from build123d import *

# Parameters (mm, degrees)
SKETCH1_W                    = 179.07
SKETCH1_H                    = 89.916
BOSS_EXTRUDE1_DEPTH          = 1.651
F_30_0_1285_DIAMETER_HOLE1_D = 3.2639
SKETCH4_W                    = 14.8844
SKETCH4_H                    = 18.8214
BOSS_EXTRUDE2_DEPTH          = 15.6718
LPATTERN1_COUNT              = 8
LPATTERN1_PITCH              = 16.4592
LPATTERN1_COUNT_DIR2         = 2
LPATTERN1_PITCH_DIR2         = 44.958
SKETCH5_W                    = 29.972
SKETCH5_H                    = 6.858
BOSS_EXTRUDE3_DEPTH          = 10.16
LPATTERN2_COUNT              = 4
LPATTERN2_PITCH              = 33.02
LPATTERN2_COUNT_DIR2         = 2
LPATTERN2_PITCH_DIR2         = 74.93
SKETCH6_W                    = 7.62
SKETCH6_H                    = 12.452922763
BOSS_EXTRUDE4_DEPTH          = 10.16
SKETCH7_W                    = 5.08
SKETCH7_H                    = 25.4
BOSS_EXTRUDE5_DEPTH          = 2.54
SKETCH8_W                    = 0.508
SKETCH8_H                    = 0.508
BOSS_EXTRUDE6_DEPTH          = 5.08
LPATTERN3_COUNT              = 10
LPATTERN3_PITCH              = 2.54
LPATTERN3_COUNT_DIR2         = 2
LPATTERN3_PITCH_DIR2         = 2.54


with BuildPart() as part:
    # Sketch1 → Boss-Extrude1 (new body)
    with BuildSketch(Plane(origin=(0, 0, 0), x_dir=(1, 0, 0), z_dir=(0, 1, 0))):
        Rectangle(SKETCH1_W, SKETCH1_H)
    extrude(amount=BOSS_EXTRUDE1_DEPTH)

    # #30 (0.1285) Diameter Hole1 (through all)
    with Locations(Plane(origin=(-85.725, 1.651, 41.021), x_dir=(0, 0, 1), z_dir=(0, 1, 0))):
        with Locations((0, 0), (-82.042, 0), (-82.042, 171.45), (0, 171.45)):
            Hole(F_30_0_1285_DIAMETER_HOLE1_D / 2)

    # Sketch4 → Boss-Extrude2 (add)
    with BuildSketch(Plane(origin=(0, 1.651, 0), x_dir=(1, 0, 0), z_dir=(0, 1, 0))):
        with Locations((-77.7494, -23.3553)):
            Rectangle(SKETCH4_W, SKETCH4_H)
    boss_extrude2 = extrude(amount=BOSS_EXTRUDE2_DEPTH)

    # LPattern1: Boss-Extrude2 8 × 2
    with Locations(*[(i * LPATTERN1_PITCH, 0, -j * LPATTERN1_PITCH_DIR2) for i in range(LPATTERN1_COUNT) for j in range(LPATTERN1_COUNT_DIR2) if (i, j) != (0, 0)]):
        add(boss_extrude2)

    # Sketch5 → Boss-Extrude3 (add)
    with BuildSketch(Plane(origin=(0, 1.651, 0), x_dir=(1, 0, 0), z_dir=(0, 1, 0))):
        with Locations((-67.945, -37.3634)):
            Rectangle(SKETCH5_W, SKETCH5_H)
    boss_extrude3 = extrude(amount=BOSS_EXTRUDE3_DEPTH)

    # LPattern2: Boss-Extrude3 4 × 2
    with Locations(*[(i * LPATTERN2_PITCH, 0, -j * LPATTERN2_PITCH_DIR2) for i in range(LPATTERN2_COUNT) for j in range(LPATTERN2_COUNT_DIR2) if (i, j) != (0, 0)]):
        add(boss_extrude3)

    # Sketch6 → Boss-Extrude4 (add)
    with BuildSketch(Plane(origin=(0, 1.651, 0), x_dir=(1, 0, 0), z_dir=(0, 1, 0))):
        with Locations((84.455, 18.157538618)):
            Rectangle(SKETCH6_W, SKETCH6_H)
    extrude(amount=BOSS_EXTRUDE4_DEPTH)

    # Sketch7 → Boss-Extrude5 (add)
    with BuildSketch(Plane(origin=(0, 1.651, 0), x_dir=(1, 0, 0), z_dir=(0, 1, 0))):
        with Locations((84.455, -4.318)):
            Rectangle(SKETCH7_W, SKETCH7_H)
    extrude(amount=BOSS_EXTRUDE5_DEPTH)

    # Sketch8 → Boss-Extrude6 (add)
    with BuildSketch(Plane(origin=(0, 4.191, 0), x_dir=(1, 0, 0), z_dir=(0, 1, 0))):
        with Locations((85.725, 7.112)):
            Rectangle(SKETCH8_W, SKETCH8_H)
    boss_extrude6 = extrude(amount=BOSS_EXTRUDE6_DEPTH)

    # LPattern3: Boss-Extrude6 10 × 2
    with Locations(*[(-j * LPATTERN3_PITCH_DIR2, 0, i * LPATTERN3_PITCH) for i in range(LPATTERN3_COUNT) for j in range(LPATTERN3_COUNT_DIR2) if (i, j) != (0, 0)]):
        add(boss_extrude6)


solid = part.part
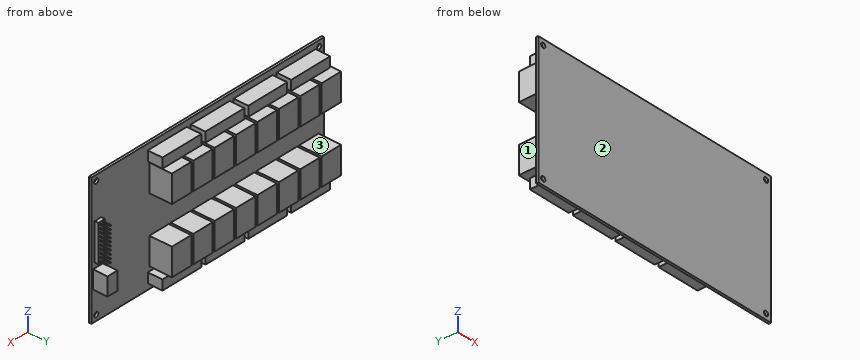
For this review, take the finished solid that the model builds, in its own axes (mm). Face numbers are marked on the shaded views. A direction names the side the tool comes from. Round coordinates to 2 decimals unless told otherwise and drop trailing zeros. Order: outer loops, then holes, each group sorted by start corner. A loop starts at its lowest first (then second) coordinate and runs counter-clockwise, first axis right, second up. Notation, with made-up numbers: M 18,4 L 45,4 A16 ccw 45,31 Z; hole C 89.5,-7.5 d3. An arc over 180 degrees is marked long. Use a Markdown table: item, result. Add a question column.
Item 1: Tool access review of the marked faces 1, 2 and 3: name each direction out of +Z, -Z, +X, -X, +Y, -Y from which nothing blocks a thin tool from reaching the whole face with its end or side.
Item 2: Add section B-B, the plane z = 37.5. Give the boundary of the cut face in (x, y) (3 decimals), then the cut area to 3 significant figures.
Item 3: Add section C-C, the plane x = 19.5. Give the boundary of the cut face in (y, z), then the cut area to 3 significant figures.
Item 4: Insertion check: pin 1 (4 mm diameter, centred on y = 5.5, z = -12, fed in from +X) (3 decimals); pin 2 (1 mm diameter, centred on x = -63.5, y = 8.5, fed in from +Z); pin 3 (0.6 mm diameter, centred on x = 83, z = -7, fed in from +Y). Each pin has a flat end and moves straight along its axis. Give the tip position at first contact, or say it passes through.
Item 5: To check wall thickness, follow line 1 along Z through (x, y) = (-81, 9.25); line 2 along X through (y, z) = (9.75, -40.5); line 3 along Z through (x, y) = (-54.5, 13.5). State the ranges of each line that lie inside material, in increasing order.
Item 6: Add section A-A, the plane y = 15. State how many separate pieces and enclosed holes the cut face has, then the cut area to 3 significant figures.
Geometry results:
| question | item | result |
|---|---|---|
| 1 | face 1 | +Z, -Z, -X, +Y |
| 1 | face 2 | +Z, -Z, +X, -X, -Y |
| 1 | face 3 | -X, +Y |
| 2 | outline | M -89.535,0 L 89.535,0 L 89.535,1.651 L 46.101,1.651 L 46.101,11.811 L 16.129,11.811 L 16.129,1.651 L 13.081,1.651 L 13.081,11.811 L -16.891,11.811 L -16.891,1.651 L -19.939,1.651 L -19.939,11.811 L -49.911,11.811 L -49.911,1.651 L -52.959,1.651 L -52.959,11.811 L -82.931,11.811 L -82.931,1.651 L -89.535,1.651 Z |
| 2 | area | 1,510 mm² |
| 3 | outline | M 0,-44.96 L 1.65,-44.96 L 1.65,-41 L 11.81,-41 L 11.81,-34.14 L 1.65,-34.14 L 1.65,-31.01 L 17.32,-31.01 L 17.32,-12.19 L 1.65,-12.19 L 1.65,13.94 L 17.32,13.94 L 17.32,32.77 L 1.65,32.77 L 1.65,33.93 L 11.81,33.93 L 11.81,40.79 L 1.65,40.79 L 1.65,44.96 L 0,44.96 Z |
| 3 | area | 878 mm² |
| 4 | pin 1 | stops at x = 88.265 |
| 4 | pin 2 | stops at z = 40.79 |
| 4 | pin 3 | stops at y = 9.27 |
| 5 | line 1 | z = -41 to -34.14, -31.01 to -12.19, 13.94 to 32.77, 33.93 to 40.79 |
| 5 | line 2 | x = -82.93 to -52.96, -49.91 to -19.94, -16.89 to 13.08, 16.13 to 46.1 |
| 5 | line 3 | z = -31.01 to -12.19, 13.94 to 32.77 |
| 6 | separate pieces | 16 |
| 6 | enclosed holes | 0 |
| 6 | area | 4,480 mm² |
